from build123d import *

# Parameters (mm, degrees)
F1_ANGLE       = 180
F4_D           = 4.5
F4_START       = 9.7071445
F4_CBORE_D     = 8
F4_CBORE_DEPTH = 8
F5_D           = 4.5
F6_DEPTH       = 16
F7_DEPTH       = 16


with BuildPart() as f1:
    # F0 (on Top) → F1 (revolve)
    with BuildSketch(Plane.XY):
        with BuildLine():
            Line((11.5, 80), (11.5, 0))
            Line((11.5, 0), (26.5, 0))
            Line((26.5, 0), (26.5, 13.8076451735))
            ThreePointArc((26.5, 13.8076451735), (25.8372883559, 16.2952001412), (24.0248281131, 18.123342452))
            ThreePointArc((24.0248281131, 18.123342452), (17.5, 29.5), (24.0248281131, 40.876657548))
            ThreePointArc((24.0248281131, 40.876657548), (25.8372883559, 42.7047998588), (26.5, 45.1923548265))
            Line((26.5, 45.1923548265), (26.5, 50.6462321396))
            ThreePointArc((26.5, 50.6462321396), (25.6700127509, 53.4050350788), (23.455602537, 55.2479295131))
            ThreePointArc((23.455602537, 55.2479295131), (17.5, 64.25), (23.455602537, 73.2520704869))
            ThreePointArc((23.455602537, 73.2520704869), (25.6700127509, 75.0949649212), (26.5, 77.8537678604))
            Line((26.5, 77.8537678604), (26.5, 80))
            Line((26.5, 80), (11.5, 80))
        make_face()
    revolve(axis=Axis((0, 49.9980136495, 0), (0, 1, 0)), revolution_arc=F1_ANGLE)

    # F4 (through all)
    # its depths count from where the whole tool has entered the part; down to there all is cleared
    with Locations(Plane(origin=(0, 0, -26.5), x_dir=(1, 0, 0), z_dir=(0, 0, -1)).offset(-F4_START)):
        with Locations((16.5, -11.5), (16.5, -48.5)):
            CounterBoreHole(F4_D / 2, F4_CBORE_D / 2, F4_CBORE_DEPTH)

    # F5 (through all)
    with Locations(Plane(origin=(0, 0, -26.5), x_dir=(1, 0, 0), z_dir=(0, 0, -1))):
        with Locations((-16.5, -48.5), (-16.5, -11.5)):
            Hole(F5_D / 2)

    # F3 (on offset) → F6 (cut)
    with BuildSketch(Plane.XY.offset(-26.5)):
        Polygon((-14.7679491924, 14.5), (-18.2320508076, 14.5), (-19.9641016151, 11.5), (-18.2320508076, 8.5), (-14.7679491924, 8.5), (-13.0358983849, 11.5), align=None)
    extrude(amount=F6_DEPTH, mode=Mode.SUBTRACT)

    # F3 (on offset) → F7 (cut)
    with BuildSketch(Plane.XY.offset(-26.5)):
        Polygon((-19.9641016151, 48.5), (-18.2320508076, 45.5), (-14.7679491924, 45.5), (-13.0358983849, 48.5), (-14.7679491924, 51.5), (-18.2320508076, 51.5), align=None)
    extrude(amount=F7_DEPTH, mode=Mode.SUBTRACT)


solid = f1.part
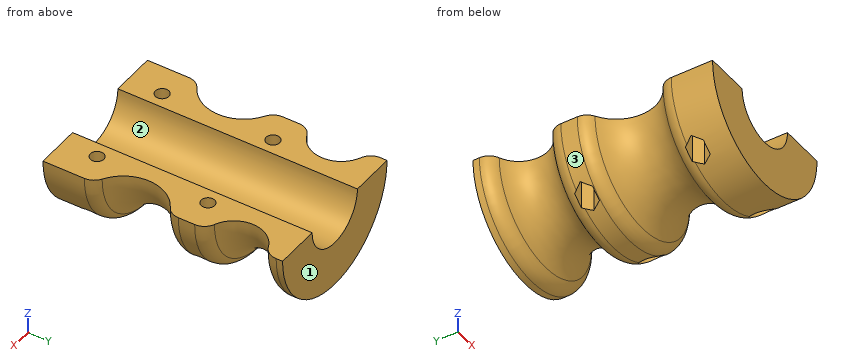
Here's how the part is built. I have some questions about the finished solid (model axes, mm). Face numbers are marked on the shaded views. Coordinates: 2 decimals unless noted, no trailing zeros. Order: outer loops, then holes, each group sorted by start corner. A loop starts at its lowest first (then second) coordinate and runs counter-clockwise, first axis right, second up. Notation, with made-up numbers: (34.5, 18) - (51.5, 18) arc R28 cw to (51.5, 49) - close; hole circle Ø4 at (84.25, 32). An arc over 180 degrees is marked (long way). Use CSV: the item, a comma, the result in double quotes. Start each with the question number.
1. Please list where these lines run through material, in increasing order: line 1 (X direction, y = 11.5, z = -5); line 2 (Y direction, x = -3, z = -21.25); line 3 (X direction, y = 48.5, z = -8). Write a range as from..to.
2. If we mould it in two halves opening along X, with no side actions, what happens to the marked faces 1, 2 and 3? For each: +X half, -X half, draft (parallel to the pull), parting line (faces both ways), or undercut.
3. Suppose I cut it at A-A on x = 0. List the corners of the cut face in (y, z) for me, then the cut area to 3 significant figures.
4. Suppose I cut it at B-B on y = 10.5. List the corners of the cut face in (x, z) for me.
5. I'm going to push flat-ended pins straight in: pin 1 (5 mm diameter, centred on x = -16.5, y = 48.5, fed in from +Z); pin 2 (8 mm diameter, centred on y = 63, z = -5.5, fed in from -X); pin 3 (9 mm diameter, centred on x = 15, y = 47, fed in from -Z); pin 4 (5 mm diameter, centred on x = 16.5, y = 11.5, fed in from -Z). Where does each tip first touch, or does it pass through?
6. Suppose I cut it at C-C on z = -6. Give the number of separate pieces and of enclosed holes in the cut face, then the cut area to 3 significant figures.
Output:
1,line 1,"x = -26.02..-18.75, -14.25..-10.36, 10.36..14.25, 18.75..26.02"
1,line 2,"y = 0..20.08, 38.92..56.39, 72.11..80"
1,line 3,"x = -25.26..-18.75, -14.25..-8.26, 8.26..14.25, 18.75..25.26"
2,face 1,"draft"
2,face 2,"undercut"
2,face 3,"parting line"
3,outline,"(0, -26.5) - (13.81, -26.5) arc R5 ccw to (18.12, -24.02) arc R13.18 cw to (40.88, -24.02) arc R5 ccw to (45.19, -26.5) - (50.65, -26.5) arc R5 ccw to (55.25, -23.46) arc R9.78 cw to (73.25, -23.46) arc R5 ccw to (77.85, -26.5) - (80, -26.5) - (80, -11.5) - (0, -11.5) - close"
3,area,"892 mm2"
4,outline,"(-26.5, 0) arc R26.5 ccw to (-19.39, -18.07) - (-19.39, -10.5) - (-18.52, -10.5) - (-18.52, 0) - close; (-14.48, -10.5) - (-13.61, -10.5) - (-13.61, -22.74) arc R26.5 ccw to (12.63, -23.3) - (12.63, -8.79) - (14.48, -8.79) - (14.48, 0) - (11.5, 0) arc R11.5 cw to (-11.5, 0) - (-14.48, 0) - close; (18.52, -8.79) - (20.37, -8.79) - (20.37, -16.95) arc R26.5 ccw to (26.5, 0) - (18.52, 0) - close"
5,pin 1,"stops at z = 0"
5,pin 2,"stops at x = -18.42"
5,pin 3,"stops at z = -24.33"
5,pin 4,"stops at z = -8.79"
6,separate pieces,"2"
6,enclosed holes,"4"
6,area,"1,860 mm2"
